For this review, take the finished solid that the model builds, in its own axes (mm). A direction names the side the tool comes from. Round coordinates to 2 decimals unless told otherwise and drop trailing zeros. Write each loop counter-clockwise with the first axis right and the second up, starting at its lowest first coordinate (ties: lowest second). Pieces come first, ordered by that corner, then holes. Notation, with made-up numbers: M 16,75.5 L 57,75.5 A23 cw 57,92.5 Z; hole C 12,10.5 d8. An arc over 180 degrees is marked long. Use one line per item in the form item = value. Start each with the question number.
Item 1: Add section D-D (y = 3.5). State the section outline as (x, z) points.
Item 2: Add section C-C (z = 23.25). State the section outline as (x, y) points.
Item 3: Add section A-A (z = 10.25). State the section outline as (x, y) points.
Item 4: Draft analysis for pull direction Y (two halves, no side actions). For faces 6 (the flat face through (27.9, 5, 12.6)), 7 (the cylindrical face through (3.01, 34.15, 2.54)), 8 (the flat face through (30, 19, 5)), 9 (the flat face through (32.1, 10, 12.6)), state which applies: released by +Y, released by -Y, zero draft, split by the parting line, or undercut.
Item 5: For line 1 (Y direction, x = 10, z = 3.2); line 2 (Z direction, x = 30, y = 7.4); line 3 (X direction, y = 29.05, z = 15), list the stretches that pass through material, from the lowest coordinate up. Write a range as [from, to].
Item 6: Add section B-B (x = 21). State the section outline as (y, z) points, and give its area (3 significant figures).
Item 7: For faces 1 (the cylindrical face through (2.85, 3.01, 2.54)), 2 (the flat face through (27.9, 32, 12.6)), 3 (the flat face through (20, 7, 10)), 4 (the flat face through (40, 8, 10)), 5 (the cylindrical face through (52.31, 9.04, 2.54)), list the 3-axis set-ups (+Z, -Z, +X, -X, +Y, -Y) from which the entire face can be reached by the end or side of a thin tool; tool diameter is ignored.
Item 8: For P1, Ø6, axis at x = 50, y = 10, coming from the +Z side; P2, Ø3, axis at x = 30, z = 15, coming from the +Y side; P3, Ø4, axis at y = 8.5, z = 10, coming from the +X side; P4, Ø10, axis at x = 26.5, z = 11, coming from the +Y side, all flat-tipped, find the tip position at first contact; note any pin that passes through.
Autodesk Inventor part; units mm, degrees
ref_plane "YZ Plane" through (0, 0, 0) normal (1, 0, 0) x (0, 1, 0)
ref_plane "XZ Plane" through (0, 0, 0) normal (0, 1, 0) x (-1, 0, 0)
ref_plane "XY Plane" through (0, 0, 0) normal (0, 0, 1) x (1, 0, 0)
sketch "Sketch1" plane through (0, 0, 0) normal (0, 0, 1) x (1, 0, 0)
  line L0 (0, 0) -> (60, 0)
  line L1 (60, 0) -> (60, 37)
  line L2 (60, 37) -> (0, 37)
  line L3 (0, 37) -> (0, 0)
  dimension "d0" = 60
  dimension "d1" = 37
extrude "Extrusion1" add sketch "Sketch1" along normal blind 5
sketch "Sketch2" plane through (0, 0, 5) normal (0, 0, 1) x (1, 0, 0)
  line L0 (20, 27) -> (40, 27)
  line L1 (40, 27) -> (40, 32)
  line L2 (40, 32) -> (20, 32)
  line L3 (20, 32) -> (20, 27)
  line L4 (20, 10) -> (40, 10)
  line L5 (40, 10) -> (40, 5)
  line L6 (40, 5) -> (20, 5)
  line L7 (20, 5) -> (20, 10)
  point P0 (0, 0)
  dimension "d6" = 20
  dimension "d7" = 5
  dimension "d8" = 20
  dimension "d9" = 5
extrude "Extrusion2" add sketch "Sketch2" along normal blind 20
sketch "Sketch3" plane through (20, 32, 5) normal (0, 1, 0) x (1, 0, 0)
  circle A0 centre (10, -10) radius 2.7
  point P0 (-20, 5)
  dimension "d12" = 5.4
extrude "Extrusion3" cut sketch "Sketch3" against normal blind 20
sketch "Sketch4" plane through (20, 10, 5) normal (0, 1, 0) x (1, 0, 0)
  circle A0 centre (10, -10) radius 2.7
  point P0 (-20, 5)
  dimension "d15" = 5.4
extrude "Extrusion4" cut sketch "Sketch4" against normal blind 20
fillet "Fillet1" radius 10 1 edges at (40, 29.5, 25)
fillet "Fillet2" radius 10 1 edges at (20, 29.5, 25)
fillet "Fillet3" radius 10 1 edges at (40, 7.5, 25)
fillet "Fillet4" radius 10 1 edges at (20, 7.5, 25)
sketch "Sketch5" plane through (0, 0, 5) normal (0, 0, 1) x (1, 0, 0)
  circle A0 centre (10, 10) radius 2.5
  circle A1 centre (50, 10) radius 2.5
  circle A2 centre (10, 27) radius 2.5
  circle A3 centre (50, 27) radius 2.5
  point P0 (0, 0)
  dimension "d22" = 5
  dimension "d23" = 5
  dimension "d24" = 5
  dimension "d25" = 5
extrude "Extrusion5" cut sketch "Sketch5" against normal blind 20
fillet "Fillet5" radius 10 1 edges at (0, 37, 2.5)
fillet "Fillet6" radius 10 1 edges at (60, 37, 2.5)
fillet "Fillet7" radius 10 1 edges at (60, 0, 2.5)
fillet "Fillet8" radius 10 1 edges at (0, 0, 2.5)
properties part number "sail_hold_1"
Calculated:
q1.outline = M 2.4,0 L 57.6,0 L 57.6,5 L 2.4,5 Z
q2.outline = M 24.35,5 L 35.65,5 L 35.65,10 L 24.35,10 Z; M 24.35,27 L 35.65,27 L 35.65,32 L 24.35,32 Z
q3.outline = M 20,5 L 40,5 L 40,10 L 20,10 Z; M 20,27 L 40,27 L 40,32 L 20,32 Z
q4.face_6 = released by -Y
q4.face_7 = released by +Y
q4.face_8 = undercut
q4.face_9 = undercut
q5.line_1 = [0, 7.5], [12.5, 24.5], [29.5, 37]
q5.line_2 = [0, 12.3], [17.7, 25]
q5.line_3 = [20, 27.3], [32.7, 40]
q6.outline = M 0,0 L 37,0 L 37,5 L 32,5 L 32,19.36 L 27,19.36 L 27,5 L 10,5 L 10,19.36 L 5,19.36 L 5,5 L 0,5 Z
q6.area = 329 mm^2
q7.face_1 = +Z, -Z, -X, -Y
q7.face_2 = +Z, +X, -X, +Y
q7.face_3 = +Z, -X, +Y, -Y
q7.face_4 = +Z, +X, +Y, -Y
q7.face_5 = +Z, -Z
q8.P1 = 5
q8.P2 = through
q8.P3 = 40
q8.P4 = 32
